Check sheet for the modelled part. Datum: model origin and axes. Units: mm. Face numbers are marked on the shaded views. A direction names the side the tool comes from. Give positions to 0.01 mm unless a question says otherwise; leave off trailing zeros. Loops run counter-clockwise (first coordinate to the right, second up) from the corner with the lowest first, then second, coordinate; pieces in that order, holes last. Notation, with made-up numbers: (52, 76) - (59, 76) arc R17 cw to (59, 104) - close; hole circle Ø4 at (45, -27). An arc over 180 degrees is marked (long way). Answer in a Markdown table with one row per item. Add a question column.
(1) Sectioned sample at C-C on y = -25. Enter the section's corners in (x, z), then the cut area to 3 significant figures.
(2) Set-up check for the marked faces 1 and 2: record each of +Z, -Z, +X, -X, +Y, -Y from which the full face is reachable in a straight line by a thin tool's end or side.
(3) Thickness scan on L1, parallel to Z at x = 30, y = -25; L2, parallel to Y at x = -27.5, z = -8; L3, parallel to X at y = -27.5, z = -18.5. Record the ranges inside material, lowest first.
(4) Sectioned sample at A-A on x = 0. Enter the section's corners in (y, z), then the cut area to 4 significant figures.
(5) Go/stop test with flat-tipped pins: P1, Ø2, axis at y = -29.5, z = -16.5, coming from the +X side; P2, Ø12, axis at x = 7.5, z = 22, coming from the +Y side; P3, Ø8, axis at y = -81, z = 8, coming from the -X side. Record where each tip stops, or that it passes through.
(6) Draft check along Y on the marked faces 3, 4 and 5. Enter one of: released by +Y, released by -Y, zero draft, split by the parting line, or undercut.
(7) Sectioned sample at D-D on x = 43. Enter the section's corners in (y, z), then the cut area to 3 significant figures.
(8) Sectioned sample at B-B on z = 0. Enter the section's corners in (x, y), then the cut area to 4 significant figures.
from build123d import *

# Parameters (mm, degrees)
F0_W     = 100
F0_H     = 100
F1_DEPTH = 65
F2_R     = 17.5
F3_DEPTH = 58
F4_SIZE  = 5
F5_R     = 21
F6_DEPTH = 25


with BuildPart() as f1:
    # F0 (on Front) → F1 (new body)
    with BuildSketch(Plane.XZ):
        Rectangle(F0_W, F0_H)
    extrude(amount=F1_DEPTH)

    # F2 (on face) → F3 (join)
    with BuildSketch(Plane.XZ.offset(65)):
        Circle(F2_R)
    extrude(amount=F3_DEPTH)

    # F4
    f4_edges = [f1.edges().sort_by_distance(p)[0] for p in [
        (50, -65, 0),
        (0, -65, -50),
        (0, -65, 50),
        (-50, -65, 0),
    ]]
    chamfer(f4_edges, length=F4_SIZE)

    # F5 (on face) → F6 (cut)
    with BuildSketch(Plane.YZ.offset(50)):
        with Locations((-25, 0)):
            Circle(F5_R)
    extrude(amount=-F6_DEPTH, mode=Mode.SUBTRACT)


solid = f1.part
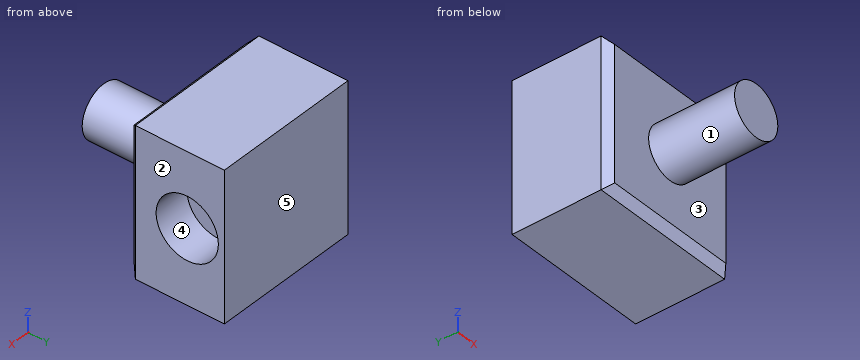
Reply:
| question | item | result |
|---|---|---|
| 1 | outline | (-50, -50) - (50, -50) - (50, -21) - (25, -21) - (25, 21) - (50, 21) - (50, 50) - (-50, 50) - close |
| 1 | area | 8,950 mm^2 |
| 2 | face 1 | -Y |
| 2 | face 2 | +Z, -Z, +X, +Y, -Y |
| 3 | L1 | -50 to -21, 21 to 50 |
| 3 | L2 | -65 to 0 |
| 3 | L3 | -50 to 25 |
| 4 | outline | (-123, -17.5) - (-65, -17.5) - (-65, -45) - (-60, -50) - (0, -50) - (0, 50) - (-60, 50) - (-65, 45) - (-65, 17.5) - (-123, 17.5) - close |
| 4 | area | 8,505 mm^2 |
| 5 | P1 | x = 25 |
| 5 | P2 | y = 0 |
| 5 | P3 | x = -17.04 |
| 6 | face 3 | released by -Y |
| 6 | face 4 | undercut |
| 6 | face 5 | released by +Y |
| 7 | outline | (-65, -45) - (-60, -50) - (0, -50) - (0, 50) - (-60, 50) - (-65, 45) - close; hole circle Ø42 at (-25, 0) |
| 7 | area | 5,090 mm^2 |
| 8 | outline | (-50, -60) - (-45, -65) - (-17.5, -65) - (-17.5, -123) - (17.5, -123) - (17.5, -65) - (45, -65) - (50, -60) - (50, -46) - (25, -46) - (25, -4) - (50, -4) - (50, 0) - (-50, 0) - close |
| 8 | area | 7,455 mm^2 |
